Input: dimensioned drawing with shaded views. Units: mm. Origin: part minimum x, y, z. A direction names the side the tool comes from. Round coordinates to 2 decimals unless told otherwise and drop trailing zeros. Loops run counter-clockwise (first coordinate to the right, second up) from the corner with the lowest first, then second, coordinate; pieces in that order, holes last. Notation, with made-up numbers: M 69,82 L 117,82 A18 ccw 117,100 Z; hole C -5.75,45 d7. An arc over 180 degrees is marked long. Write each question's results on one line, items separated by ' | '. Start each with the question number.
1. Set-up query: the marked faces 4 and 5. Return all of +Z, -Z, +X, -X, +Y, -Y with unobstructed straight access to the full face (end or side cutting, diameter ignored); none if empty.
2. Ray query, line 1 (Y direction, x = 23.5, z = 20.5); line 2 (Z direction, x = 16, y = 7); line 3 (Y direction, x = 3, z = 4.5). Return the intervals inside material, ascending.
3. Section B-B on z = 4.5. Output: boundary loops of the cut face in (x, y).
4. Section A-A on x = 25. Output: boundary loops of the cut face in (y, z), and give its area (3 significant figures).
5. Section D-D on x = 4. Output: boundary loops of the cut face in (y, z), and give its area (3 significant figures).
6. Draft query along Z for the marked faces 1, 2 and 3. Return one class per face: released by +Z, released by -Z, zero draft, split by the parting line, or undercut.
7. Section C-C on y = 6. Output: boundary loops of the cut face in (x, z).
8. Contact query for flat-ended pins moving along their axis: pin 1 Ø4 at (x, y) = (35.5, 5.5) entering from -Z; pin 2 Ø5 at (x, z) = (41.5, 30.5) entering from -Y; pin 3 Ø17.5 at (x, z) = (37, 28.5) entering from +Y. Output: stop coordinate, or through.
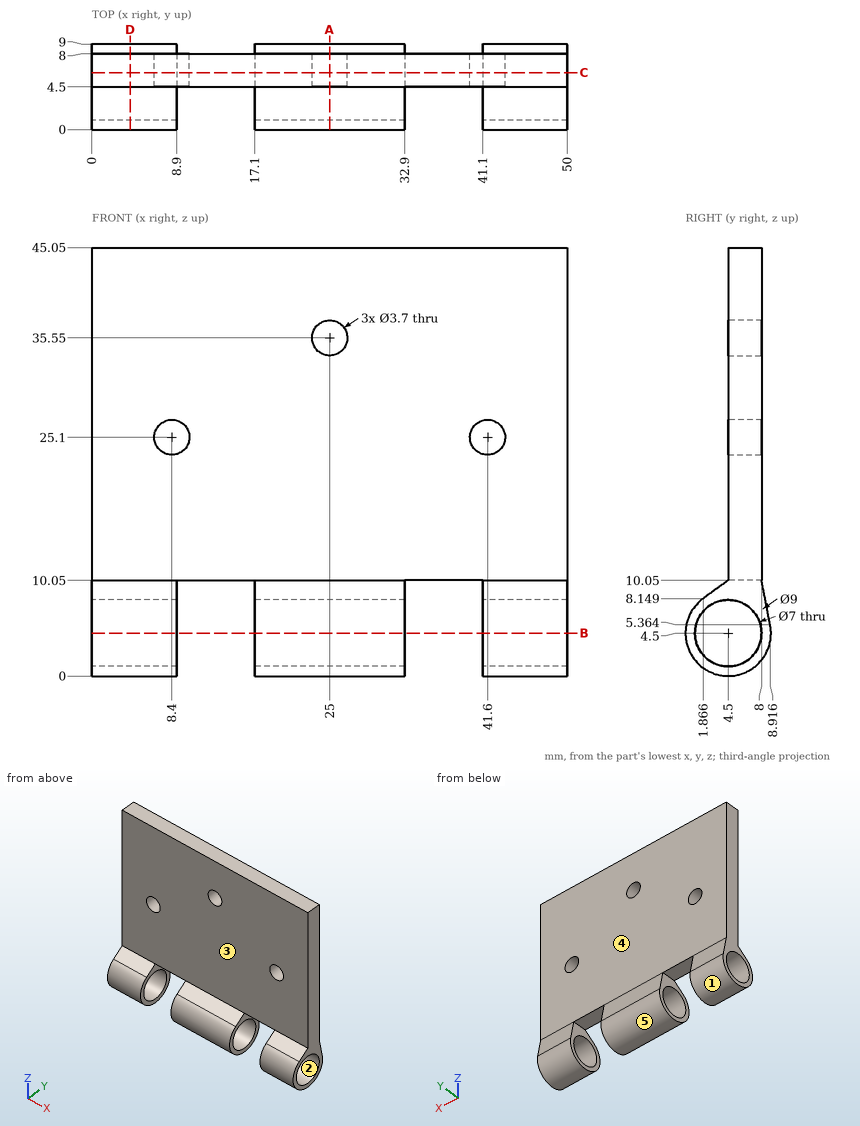
Taken from the geometry:
1) face 4: +Z, +X, -X, +Y | face 5: +X, -X
2) line 1: 4.5 to 8 | line 2: 10.05 to 45.05 | line 3: 0 to 1, 8 to 9
3) outline: M 0,0 L 8.9,0 L 8.9,1 L 0,1 Z; M 0,8 L 8.9,8 L 8.9,9 L 0,9 Z; M 17.1,0 L 32.9,0 L 32.9,1 L 17.1,1 Z; M 17.1,8 L 32.9,8 L 32.9,9 L 17.1,9 Z; M 41.1,0 L 50,0 L 50,1 L 41.1,1 Z; M 41.1,8 L 50,8 L 50,9 L 41.1,9 Z
4) outline: M 1.87,8.15 A4.5 ccw long 8.92,5.36 L 8,10.05 L 8,33.7 L 4.5,33.7 L 4.5,10.05 Z; M 4.5,37.4 L 8,37.4 L 8,45.05 L 4.5,45.05 Z; hole C 4.5,4.5 d7 | area: 142 mm^2
5) outline: M 1.87,8.15 A4.5 ccw long 8.92,5.36 L 8,10.05 L 8,45.05 L 4.5,45.05 L 4.5,10.05 Z; hole C 4.5,4.5 d7 | area: 155 mm^2
6) face 1: split by the parting line | face 2: undercut | face 3: zero draft
7) outline: M 0,0.26 L 8.9,0.26 L 8.9,1.34 L 0,1.34 Z; M 0,7.66 L 8.9,7.66 L 8.9,10.05 L 17.1,10.05 L 17.1,7.66 L 32.9,7.66 L 32.9,10.05 L 41.1,10.05 L 41.1,7.66 L 50,7.66 L 50,45.05 L 0,45.05 Z; M 17.1,0.26 L 32.9,0.26 L 32.9,1.34 L 17.1,1.34 Z; M 41.1,0.26 L 50,0.26 L 50,1.34 L 41.1,1.34 Z; hole C 8.4,25.1 d3.7; hole C 25,35.55 d3.7; hole C 41.6,25.1 d3.7
8) pin 1: z = 10.05 | pin 2: y = 4.5 | pin 3: y = 8
